Can you work these out from the model? Positions are in its coordinate system, mm. A direction names the side the tool comes from. Round coordinates to 2 decimals unless told otherwise and drop trailing zeros. Order: outer loops, then holes, each group sorted by start corner. A loop starts at its lowest first (then second) coordinate and runs counter-clockwise, first axis right, second up. Notation, with made-up numbers: (-25.75, 20) -> (19.25, 20) arc R23 cw to (19.25, 56) -> close; hole circle Ø6 at (84.5, 71.25). An arc over 180 degrees is marked (long way). Use a Markdown table: item, result. Add a question column.
Q1. If we section it at D-D on z = 7.75: List the corners of the cut face in (x, y) for me (1 decimal).
Q2. If we section it at B-B on x = -12: List the corners of the cut face in (y, z) for me, plus the area to 3 significant figures.
Q3. For faces 1 (the face through (0, 3.507, 4)), 2 (the face through (17.8, -2.78, 0.83)), 3 (the face through (0, 4, 5.486)), which set-ups out of +Z, -Z, +X, -X, +Y, -Y let a thin tool reach every point of the face, with its end or its side?
Q4. If we section it at C-C on y = 0: List the corners of the cut face in (x, z) for me (3 decimals), plus the area to 3 significant figures.
Q5. We'd pull the mould along Y, two halves only. Please class faces 4 (the face through (26.504, 1.73, 0.826)), 5 (the face through (0, -4.636, 5)), 6 (the face through (-33.655, 0.3, 1.5)), 7 (the face through (0, 0, 1.676)): +Y half, -Y half, draft (parallel to the pull), parting line (faces both ways), or undercut.
Q6. I need wall thicknesses on line 1 along Y through (x, z) = (-3, 4.75); line 2 along X through (y, z) = (-2.5, 1) (3 decimals); line 3 along Z through (x, y) = (-9.5, -2). Which ranges of each line are inside material? Lowest first, please. Write a range as [from, to].
Q7. If we section it at A-A on z = 4.25: List the corners of the cut face in (x, y) for me (1 decimal).
Q8. I'm going to push flat-ended pins straight in: pin 1 Ø0.9 at (x, y) = (-14.5, 4) entering from +Z; pin 2 Ø3.5 at (x, y) = (12.5, 1.5) entering from +Z; pin 3 Ø1 at (x, z) = (-25, 8) entering from +Y; pin 4 Ø0.8 at (x, y) = (25.89, -2.35) entering from -Z. Where does each tip first touch, or does it pass through?
```python
from build123d import *

# Parameters (mm, degrees)
F0_W     = 67.564
F0_H     = 9.271
F1_DEPTH = 1.6764
F2_W     = 67.564
F2_H     = 1.11254
F3_DEPTH = 7.62
F2_H_2   = 1.128524
F4_DEPTH = 3.81
F5_R     = 0.638652
F5_R_2   = 0.640447
F5_R_3   = 0.63486
F5_R_4   = 0.631082
F6_DEPTH = 25.4


with BuildPart() as f1:
    # F0 (on Top) → F1 (new body)
    with BuildSketch(Plane.XY):
        with Locations((0.127, 0)):
            Rectangle(F0_W, F0_H)
    extrude(amount=F1_DEPTH)

    # F2 (on face) → F3 (join)
    with BuildSketch(Plane.XY.offset(1.6764)):
        with Locations((0.127, -4.07923)):
            Rectangle(F2_W, F2_H)
    extrude(amount=F3_DEPTH)

    # F2 (on face) → F4 (join)
    with BuildSketch(Plane.XY.offset(1.6764)):
        with Locations((0.127, 4.071238)):
            Rectangle(F2_W, F2_H_2)
    extrude(amount=F4_DEPTH)

    # F5 (on face) → F6 (cut)
    with BuildSketch(Plane(origin=(0, 0, 0), x_dir=(1, 0, 0), z_dir=(0, 0, -1))):
        with Locations((25.892904, 2.352488)):
            Circle(F5_R)
        with Locations((25.892904, -1.9222)):
            Circle(F5_R_2)
        with Locations((18.270466, 2.352488)):
            Circle(F5_R_3)
        with Locations((18.270466, -1.9222)):
            Circle(F5_R_4)
    extrude(amount=-F6_DEPTH, mode=Mode.SUBTRACT)


solid = f1.part
```
Answer below:
| question | item | result |
|---|---|---|
| 1 | outline | (-33.7, -4.6) -> (33.9, -4.6) -> (33.9, -3.5) -> (-33.7, -3.5) -> close |
| 2 | outline | (-4.64, 0) -> (4.64, 0) -> (4.64, 5.49) -> (3.51, 5.49) -> (3.51, 1.68) -> (-3.52, 1.68) -> (-3.52, 9.3) -> (-4.64, 9.3) -> close |
| 2 | area | 28.3 mm² |
| 3 | face 1 | +Z, +X, -X |
| 3 | face 2 | +Z, -Z |
| 3 | face 3 | +Z, +X, -X, +Y |
| 4 | outline | (-33.655, 0) -> (33.909, 0) -> (33.909, 1.676) -> (-33.655, 1.676) -> close |
| 4 | area | 113 mm² |
| 5 | face 4 | undercut |
| 5 | face 5 | -Y half |
| 5 | face 6 | draft |
| 5 | face 7 | undercut |
| 6 | line 1 | [-4.64, -3.52], [3.51, 4.64] |
| 6 | line 2 | [-33.655, 17.653], [18.888, 25.272], [26.514, 33.909] |
| 6 | line 3 | [0, 1.68] |
| 7 | outline | (-33.7, -4.6) -> (33.9, -4.6) -> (33.9, -3.5) -> (-33.7, -3.5) -> close; (-33.7, 3.5) -> (33.9, 3.5) -> (33.9, 4.6) -> (-33.7, 4.6) -> close |
| 8 | pin 1 | z = 5.49 |
| 8 | pin 2 | z = 1.68 |
| 8 | pin 3 | y = -3.52 |
| 8 | pin 4 | through |
